Design review of the part built by this model. Coordinates are the model's own, in mm. Round coordinates to 2 decimals unless told otherwise and drop trailing zeros. Loops run counter-clockwise (first coordinate to the right, second up) from the corner with the lowest first, then second, coordinate; pieces in that order, holes last. Notation, with made-up numbers: (16.25, 89.25) - (34.25, 89.25) arc R36 cw to (34.25, 125.25) - close; hole circle Ø2 at (13, 73). An arc over 180 degrees is marked (long way). Return JSON: item names as keys, results as strings. Group by question number.
(1) Wall thickness on L1, parallel to Z at x = 379, y = -2.25; L2, parallel to X at y = -1.25, z = 50; L3, parallel to X at y = -6.5, z = 49: over which ranges is each line inside the solid? List them lowest first. Write a range as [from, to].
(2) Clearance check with flat-ended pins moving along their axes: pin 1 (2 mm diameter, centred on y = -2.5, z = 49, fed in from +X); pin 2 (4 mm diameter, centred on y = -6, z = 48, fed in from -X); pin 3 (1.5 mm diameter, centred on y = -5, z = 57.5, fed in from -X). State where each tip first meets the part, or that it passes through.
(3) We need section A-A, the plane x = 962. Write out the cut boundary in (y, z), and give its area (3 significant figures).
(4) We need section B-B, the plane z = 31.5. Write out the cut boundary in (x, y).
from build123d import *

# Parameters (mm, degrees)
F1_DEPTH = 7.112
F3_DEPTH = 25.4
F6_DEPTH = 25.4


with BuildPart() as f1:
    # F0 (on Front) → F1 (new body)
    with BuildSketch(Plane.XZ):
        with BuildLine():
            Line((-134.4452477908, 13.9205330778), (1389.5547522092, 13.9205330778))
            ThreePointArc((1389.5547522092, 13.9205330778), (1422.5747522092, 46.9405330778), (1389.5547522092, 79.9605330778))
            Line((1389.5547522092, 79.9605330778), (-134.4452477908, 79.9605330778))
            ThreePointArc((-134.4452477908, 79.9605330778), (-167.4652477908, 46.9405330778), (-134.4452477908, 13.9205330778))
        make_face()
        with BuildLine():
            ThreePointArc((-134.4452477908, 16.4605330778), (-164.9252477908, 46.9405330778), (-134.4452477908, 77.4205330778))
            Line((-134.4452477908, 77.4205330778), (1389.5547522092, 77.4205330778))
            ThreePointArc((1389.5547522092, 77.4205330778), (1420.0347522092, 46.9405330778), (1389.5547522092, 16.4605330778))
            Line((1389.5547522092, 16.4605330778), (-134.4452477908, 16.4605330778))
        make_face(mode=Mode.SUBTRACT)
    extrude(amount=F1_DEPTH)

    # F2 (on face) → F3 (cut)
    with BuildSketch(Plane.XY.offset(79.9605330778)):
        with BuildLine():
            Line((28.1147522092, -4.6345466567), (28.1147522092, -2.4774533433))
            ThreePointArc((28.1147522092, -2.4774533433), (27.0362055525, -3.556), (28.1147522092, -4.6345466567))
        make_face()
        with BuildLine():
            ThreePointArc((29.1932988659, -3.556), (28.877399864, -2.7933523452), (28.1147522092, -2.4774533433))
            Line((28.1147522092, -2.4774533433), (28.1147522092, -4.6345466567))
            ThreePointArc((28.1147522092, -4.6345466567), (28.877399864, -4.3186476548), (29.1932988659, -3.556))
        make_face()
    extrude(amount=-F3_DEPTH, mode=Mode.SUBTRACT)

    # F5 (on face) → F6 (cut)
    with BuildSketch(Plane(origin=(0, 0, 13.9205330778), x_dir=(1, 0, 0), z_dir=(0, 0, -1))):
        with BuildLine():
            ThreePointArc((-134.4452477908, 2.2867995466), (-133.5477875436, 2.6585397527), (-133.1760473375, 3.556))
            ThreePointArc((-133.1760473375, 3.556), (-133.5477875436, 4.4534602473), (-134.4452477908, 4.8252004534))
            Line((-134.4452477908, 4.8252004534), (-134.4452477908, 2.2867995466))
        make_face()
        with BuildLine():
            Line((-134.4452477908, 2.2867995466), (-134.4452477908, 4.8252004534))
            ThreePointArc((-134.4452477908, 4.8252004534), (-135.7144482442, 3.556), (-134.4452477908, 2.2867995466))
        make_face()
    extrude(amount=-F6_DEPTH, mode=Mode.SUBTRACT)


solid = f1.part
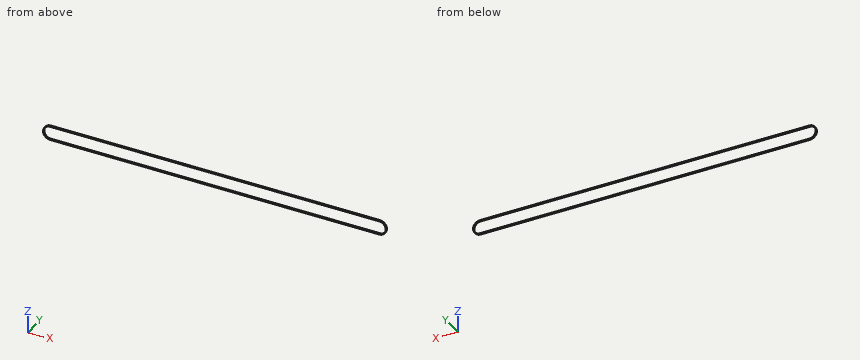
Solutions:
{
 "1": {"L1": "[13.92, 16.46], [77.42, 79.96]", "L2": "[-167.32, -164.77], [1419.88, 1422.43]", "L3": "[-167.4, -164.86], [1419.97, 1422.51]"},
 "2": {"pin 1": "x = 1422.56", "pin 2": "x = -167.47", "pin 3": "x = -165.97"},
 "3": {"outline": "(-7.11, 13.92) - (0, 13.92) - (0, 16.46) - (-7.11, 16.46) - close; (-7.11, 77.42) - (0, 77.42) - (0, 79.96) - (-7.11, 79.96) - close", "area": "36.1 mm^2"},
 "4": {"outline": "(-163.63, -7.11) - (-160.72, -7.11) - (-160.72, 0) - (-163.63, 0) - close; (1415.83, -7.11) - (1418.74, -7.11) - (1418.74, 0) - (1415.83, 0) - close"}
}
